Verification items for this drawing (mm, ordinates from the low corner). A direction names the side the tool comes from. Coordinates: 2 decimals unless noted, no trailing zeros. Write each loop counter-clockwise with the first axis right and the second up, starting at its lowest first coordinate (ties: lowest second). Pieces come first, ordered by that corner, then holes. Notation, with made-up numbers: (-18, 11) -> (8, 11) arc R22 ccw to (8, 41) -> close; hole circle Ø6 at (-38.5, 18). An arc over 180 degrees is marked (long way). One line per item, written item: value. Start each with the question number.
1) Sectioned sample at D-D on z = 30. Enter the section's corners in (x, y), plus the area to 3 significant figures.
2) Sectioned sample at C-C on x = 8.5. Enter the section's corners in (y, z).
3) Scan lines: line 1 along X through (y, z) = (40.5, 32.5); line 2 along Y through (x, z) = (50, 32); line 3 along Y through (x, z) = (24, 31.5). Record each from-to range of solid material in increasing order. Write a range as [from, to].
4) Set-up check for the marked faces 1 and 2: record each of +Z, -Z, +X, -X, +Y, -Y from which the full face is reachable in a straight line by a thin tool's end or side.
5) Gauge pin test, flat ends, axial feed: P1, Ø12, axis at y = 48.5, z = 25, coming from the +X side; P2, Ø5, axis at x = 28, z = 11, coming from the +Y side; P3, Ø1.5, axis at x = 7, y = 41, coming from the -Z side; P4, Ø1, axis at x = 8, z = 4, coming from the +Y side. Record the tip position at first contact, or that the pin passes through.
6) Sectioned sample at B-B on z = 6.5. Enter the section's corners in (x, y).
7) Sectioned sample at A-A on z = 20. Enter the section's corners in (x, y), plus the area to 4 significant figures.
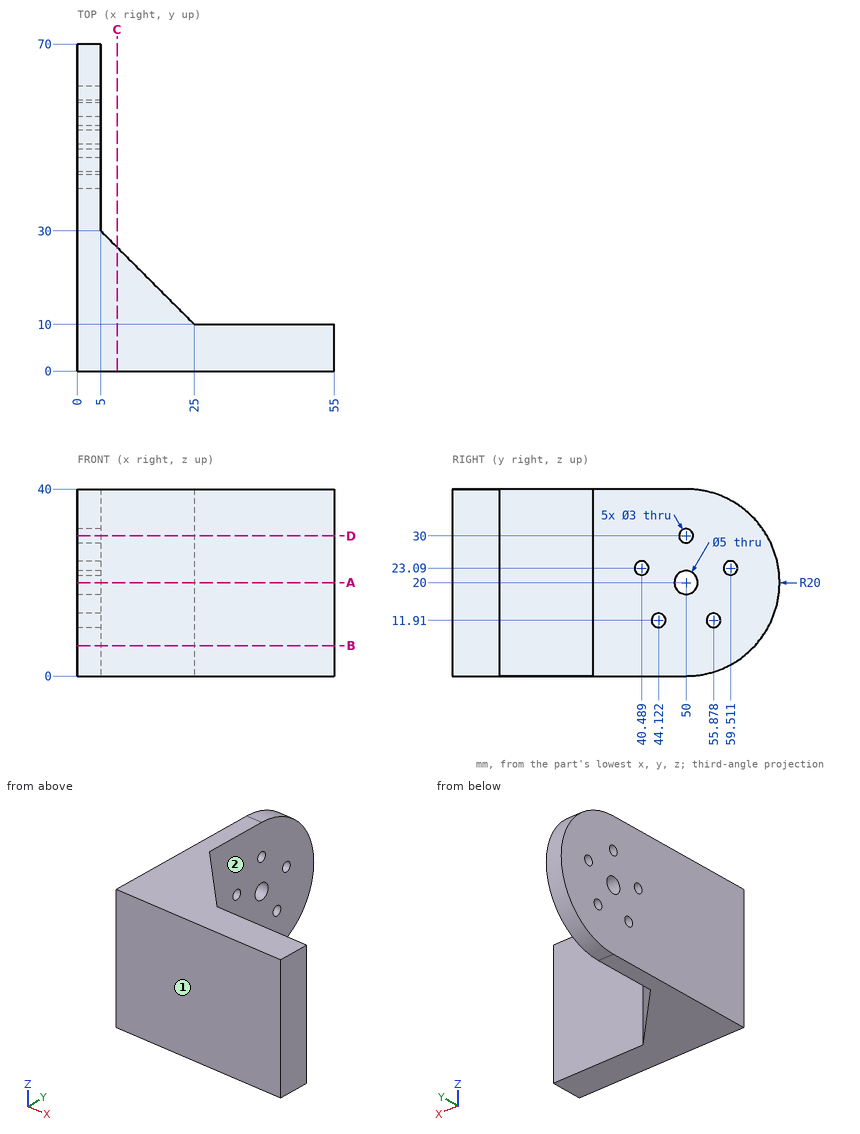
Answers:
1. outline: (0, 0) -> (55, 0) -> (55, 10) -> (25, 10) -> (5, 30) -> (5, 48.5) -> (0, 48.5) -> close; (0, 51.5) -> (5, 51.5) -> (5, 67.32) -> (0, 67.32) -> close
1. area: 1,020 mm2
2. outline: (0, 0) -> (26.5, 0) -> (26.5, 40) -> (0, 40) -> close
3. line 1: x = [0, 5]
3. line 2: y = [0, 10]
3. line 3: y = [0, 11]
4. face 1: +Z, -Z, +X, -X, -Y
4. face 2: +Z, -Z, +X, +Y
5. P1: stops at x = 5
5. P2: stops at y = 10
5. P3: passes through
5. P4: stops at y = 27.5
6. outline: (0, 0) -> (55, 0) -> (55, 10) -> (25, 10) -> (5, 30) -> (5, 64.76) -> (0, 64.76) -> close
7. outline: (0, 0) -> (55, 0) -> (55, 10) -> (25, 10) -> (5, 30) -> (5, 47.5) -> (0, 47.5) -> close; (0, 52.5) -> (5, 52.5) -> (5, 70) -> (0, 70) -> close
7. area: 1,025 mm2
